The model under review builds one solid part; all positions refer to its coordinate system, in mm. A direction names the side the tool comes from. Round coordinates to 2 decimals unless told otherwise and drop trailing zeros. Write each loop counter-clockwise with the first axis right and the second up, starting at its lowest first coordinate (ties: lowest second). Pieces come first, ordered by that corner, then holes.
Item 1: Clearance check with flat-ended pins moving along their axes: pin 1 Ø1.4 at (x, y) = (6, 5) entering from -Z; pin 2 Ø1 at (x, z) = (21, 0.5) entering from +Y; pin 3 Ø4 at (x, y) = (83.5, 4) entering from -Z; pin 4 Ø3 at (x, y) = (17, 3.5) entering from -Z. State where each tip first meets the part, or that it passes through.
Item 2: Draft analysis for pull direction X (two halves, no side actions). For faces 1 (the face through (89.321, 4.93, 0.465)), 2 (the face through (69, 3, -2.8)), 3 (the face through (19.43, 1.67, -1.79)), state which applies: +X half, -X half, draft (parallel to the pull), parting line (faces both ways), or undercut.
Item 3: To check wall thickness, follow L1, parallel to Y at x = 15, z = 8; L2, parallel to X at y = 4.5, z = 1.5; L3, parallel to X at y = 4, z = 4. State the ranges of each line that lie inside material, in increasing order.
Item 4: Machinability: for faces 4 (the face through (22, 9, 1.2)), 5 (the face through (80.5, 5, -1)), 6 (the face through (77.347, 5.103, 6.131)), which of the approach directions +Z, -Z, +X, -X, +Y, -Y give a long, thin tool a straight path to every point of the face, cutting with its end or side? Answer none if there is none.
Item 5: Add section D-D (x = 45). Give the boundary of the cut face in (y, z), plus the area to 3 significant figures.
Item 6: Add section B-B (z = 7.75). Give the boundary of the cut face in (x, y), plus the area to 3 significant figures.
Item 7: Add section C-C (y = 8.75). Give the boundary of the cut face in (x, z), plus the area to 3 significant figures.
Item 8: Add section A-A (x = 75). Give the boundary of the cut face in (y, z).
```python
from build123d import *
from OCP.BRepFilletAPI import BRepFilletAPI_MakeChamfer

# Parameters (mm, degrees)
SKETCH2_W                       = 90
SKETCH2_H                       = 10
BOSS_EXTRUDE1_DEPTH             = 9.35
SKETCH4_W                       = 9.5
SKETCH4_H                       = 10
BOSS_EXTRUDE2_DEPTH             = 2
SKETCH5_R                       = 1.45
BOSS_EXTRUDE3_DEPTH             = 2.8
CHAMFER1_SIZE                   = 0.8
CHAMFER2_SIZE                   = 5
CHAMFER2_SIZE2                  = 1.339745962
F_13_0_185_DIAMETER_HOLE1_D     = 4.699
F_13_0_185_DIAMETER_HOLE1_DEPTH = 6.35
F_6_CLEARANCE_HOLE1_D           = 3.7973
F_6_CLEARANCE_HOLE1_ON_FACE_2_D = 3.7973
F_13_0_185_DIAMETER_HOLE2_D     = 4.699
F_13_0_185_DIAMETER_HOLE2_DEPTH = 6.35
F_6_CLEARANCE_HOLE2_D           = 3.7973
CUT_EXTRUDE1_DEPTH              = 92.035281622
CUT_EXTRUDE1_DEPTH_BACK         = 1.2
SKETCH12_W                      = 28.5
SKETCH12_H                      = 10
SKETCH12_W_2                    = 5.2
SKETCH12_H_2                    = 2
SKETCH12_W_3                    = 2.7
SKETCH12_H_3                    = 0.5


with BuildPart() as part:
    # Sketch2 → Boss-Extrude1 (new body)
    with BuildSketch(Plane.XY):
        with Locations((45, 5)):
            Rectangle(SKETCH2_W, SKETCH2_H)
    extrude(amount=BOSS_EXTRUDE1_DEPTH)

    # Sketch4 → Boss-Extrude2 (add)
    with BuildSketch(Plane(origin=(0, 0, 0), x_dir=(-1, 0, 0), z_dir=(0, 0, -1))):
        with Locations((-4.75, 5)):
            Rectangle(SKETCH4_W, SKETCH4_H)
        with Locations((-85.25, 5)):
            Rectangle(SKETCH4_W, SKETCH4_H)
    extrude(amount=BOSS_EXTRUDE2_DEPTH)

    # Sketch5 → Boss-Extrude3 (add)
    with BuildSketch(Plane(origin=(0, 0, 0), x_dir=(-1, 0, 0), z_dir=(0, 0, -1))):
        with Locations(Location((-69.137406388, 2.998839673, 0), (0, 0, 180))):
            Circle(SKETCH5_R)
        with Locations(Location((-20.877406388, 1.728839673, 0), (0, 0, 180))):
            Circle(SKETCH5_R)
    extrude(amount=BOSS_EXTRUDE3_DEPTH)

    # Chamfer1
    # the kernel refuses this chamfer: 0.8 mm, written as the material it adds along each edge
    with BuildSketch(Plane(origin=(69.137406388, 2.998839673, 0), x_dir=(1, 0, 0), z_dir=(0, 1, 0))) as chamfer1_piece_1:
        Polygon((1.45 + CHAMFER1_SIZE, 0), (1.45, CHAMFER1_SIZE), (1.45, 0), align=None)
    revolve(axis=Axis((69.137406388, 2.998839673, 0), (0, 0, -1)))
    with BuildSketch(Plane(origin=(20.877406388, 1.728839673, 0), x_dir=(1, 0, 0), z_dir=(0, 1, 0))) as chamfer1_piece_2_section:
        Polygon((1.45 + CHAMFER1_SIZE, 0), (1.45, CHAMFER1_SIZE), (1.45, 0), align=None)
    chamfer1_piece_2 = revolve(axis=Axis((20.877406388, 1.728839673, 0), (0, 0, -1)), mode=Mode.PRIVATE)
    chamfer1_piece_2 = split(chamfer1_piece_2, bisect_by=Plane(origin=(19.038199604, 0, -0.389206784), z_dir=(0, 1, 0)), keep=Keep.TOP, mode=Mode.PRIVATE)
    add(chamfer1_piece_2)

    # Chamfer2: one chamfer whose edges measure the first distance from different faces: ONE call of the kernel's chamfer builder (chamfer() names one face for all edges)
    chamfer2_edges_1 = [part.edges().sort_by_distance(p)[0] for p in [
        (0, 5, -2),
    ]]
    chamfer2_side_1 = [part.faces().sort_by_distance(p)[0] for p in [
        (0, 5, 3.675),
    ]]
    chamfer2_edges_2 = [part.edges().sort_by_distance(p)[0] for p in [
        (90, 5, -2),
    ]]
    chamfer2_side_2 = [part.faces().sort_by_distance(p)[0] for p in [
        (90, 5, 3.675),
    ]]
    chamfer2 = BRepFilletAPI_MakeChamfer(part.part.solid().wrapped)
    for e in chamfer2_edges_1:
        chamfer2.Add(CHAMFER2_SIZE, CHAMFER2_SIZE2, e.wrapped, chamfer2_side_1[0].wrapped)  # the first distance lies on this face
    for e in chamfer2_edges_2:
        chamfer2.Add(CHAMFER2_SIZE, CHAMFER2_SIZE2, e.wrapped, chamfer2_side_2[0].wrapped)  # the first distance lies on this face
    add(Compound.cast(chamfer2.Shape()), mode=Mode.REPLACE)

    # #13 (0.185) Diameter Hole1
    with Locations(Plane(origin=(84.580127019, 5, -2), x_dir=(-1, 0, 0), z_dir=(0, 0, -1))):
        with Locations((0, 0), (79.160254038, 0)):
            Hole(F_13_0_185_DIAMETER_HOLE1_D / 2, depth=F_13_0_185_DIAMETER_HOLE1_DEPTH)

    # #6 Clearance Hole1 (through all)
    with Locations(Plane(origin=(84.580127019, 5, 4.35), x_dir=(-1, 0, 0), z_dir=(0, 0, -1))):
        with Locations((0, 0), (79.160254038, 0)):
            Hole(F_6_CLEARANCE_HOLE1_D / 2)

    # #6 Clearance Hole1 on face 2 (through all)
    with Locations(Plane(origin=(5.419872981, 5, 0), x_dir=(-1, 0, 0), z_dir=(0, 0, -1))):
        with Locations((0, 0)):
            Hole(F_6_CLEARANCE_HOLE1_ON_FACE_2_D / 2)

    # #13 (0.185) Diameter Hole2
    with Locations(Plane(origin=(75, 5, 9.35), x_dir=(1, 0, 0), z_dir=(0, 0, 1))):
        with Locations((0, 0), (-60, 0)):
            Hole(F_13_0_185_DIAMETER_HOLE2_D / 2, depth=F_13_0_185_DIAMETER_HOLE2_DEPTH)

    # #6 Clearance Hole2 (through all)
    with Locations(Plane(origin=(75, 5, 3), x_dir=(1, 0, 0), z_dir=(0, 0, 1))):
        with Locations((0, 0), (-60, 0)):
            Hole(F_6_CLEARANCE_HOLE2_D / 2)

    # Sketch12 → Cut-Extrude1 (cut, two sides: drawn at the far end of the back side and taken through both)
    with BuildSketch(Plane(origin=(0, 0, 0), x_dir=(-1, 0, 0), z_dir=(0, 0, -1)).offset(-CUT_EXTRUDE1_DEPTH_BACK)):
        with Locations((-40.75, 5)):
            Rectangle(SKETCH12_W, SKETCH12_H)
        with Locations((-21.7, 9)):
            Rectangle(SKETCH12_W_2, SKETCH12_H_2)
        with Locations((-69.15, 0.25)):
            Rectangle(SKETCH12_W_3, SKETCH12_H_3)
    extrude(amount=CUT_EXTRUDE1_DEPTH + CUT_EXTRUDE1_DEPTH_BACK, mode=Mode.SUBTRACT)


solid = part.part
```
Numbers:
1. pin 1: passes through
1. pin 2: stops at y = 8
1. pin 3: stops at z = -2
1. pin 4: stops at z = 0
2. face 1: +X half
2. face 2: draft
2. face 3: undercut
3. L1: y = 0 to 2.65, 7.35 to 10
3. L2: x = 0.4 to 3.12, 7.72 to 13.17, 16.83 to 73.17, 76.83 to 82.28, 86.88 to 89.6
3. L3: x = 0 to 3.29, 7.55 to 12.87, 17.13 to 72.87, 77.13 to 82.45, 86.71 to 90
4. face 4: -Z, +Y
4. face 5: -Z, +Y, -Y
4. face 6: +Z
5. outline: (0, 1.2) - (10, 1.2) - (10, 9.35) - (0, 9.35) - close
5. area: 81.5 mm2
6. outline: (0, 0) - (90, 0) - (90, 10) - (0, 10) - close; hole circle Ø3.8 at (5.42, 5); hole circle Ø4.7 at (15, 5); hole circle Ø4.7 at (75, 5); hole circle Ø3.8 at (84.58, 5)
6. area: 843 mm2
7. outline: (0, 3) - (1.34, -2) - (9.5, -2) - (9.5, 0) - (19.1, 0) - (19.1, 1.2) - (24.3, 1.2) - (24.3, 0) - (26.5, 0) - (26.5, 1.2) - (55, 1.2) - (55, 0) - (80.5, 0) - (80.5, -2) - (88.66, -2) - (90, 3) - (90, 9.35) - (0, 9.35) - close
7. area: 832 mm2
8. outline: (0, 0) - (3.1, 0) - (3.1, 3) - (2.65, 3) - (2.65, 9.35) - (0, 9.35) - close; (6.9, 0) - (10, 0) - (10, 9.35) - (7.35, 9.35) - (7.35, 3) - (6.9, 3) - close
